```python
from build123d import *

# Parameters (mm, degrees)
F1_R = 6.35


with BuildPart() as f2:
    # F2: sweep along a path in F0
    with BuildLine(Plane.XZ) as f2_path:
        Line((-51.7302755781, 114.3), (-34.3931889452, 140.4537514452))
        ThreePointArc((-34.3931889452, 140.4537514452), (-43.0445729181, 164.4248458133), (-63.5, 149.225))
        Line((-63.5, 149.225), (-63.5, -19.05))
        ThreePointArc((-63.5, -19.05), (-31.75, -50.8), (0, -19.05))
        Line((0, -19.05), (0, 0))
    # F1 (on Top) → F2 (sweep)
    with BuildSketch(Plane.XY):
        Circle(F1_R)
    sweep(path=f2_path.line)


solid = f2.part
```
Build history of the part. All positions in model axes, mm. Coordinates: 2 decimals unless noted, no trailing zeros. Order: outer loops, then holes, each group sorted by start corner. A loop starts at its lowest first (then second) coordinate and runs counter-clockwise, first axis right, second up. Notation, with made-up numbers: (20, 4.5) -> (62, 4.5) arc R18 ccw to (62, 31.5) -> close; hole circle Ø7 at (48, 1.5). An arc over 180 degrees is marked (long way). Answer in a Markdown table with one row per item. Add a question column.
Q1. Band-saw the part on A-A, the plane z = 55. List the corners of the cut face in (x, y).
Q2. Drop flat-ended pins along their axis: pin 1 (1.5 mm diameter, centred on y = 3, z = 81.5, fed in from -X); pin 2 (4 mm diameter, centred on y = 4, z = 59.5, fed in from -X); pin 3 (2 mm diameter, centred on x = -43, y = -3.5, fed in from -Z). Give the stop position or say it passes through.
Q3. Band-saw the part on C-C, the plane x = -42. Give the number of separate pieces and of enclosed holes in the cut face, then the cut area to 3 significant figures.
Q4. Mould opens along Z. For faces 1 (the face through (-48.228, 0.279, 131.065)), 2 (the face through (0, 0, 0)), 3 (the face through (-51.804, 0.089, 114.349)), 4 (the face through (6.057, 1.907, -9.392)) say: +Z half, -Z half, draft (parallel to the pull), parting line (faces both ways), or undercut.
Q5. Wall check: line 1 along Z through (x, y) = (-53, -2.5); line 2 along Z through (x, y) = (-32, 4.5); line 3 along X through (y, z) = (0, 92.5). Give the ranges that are in metal, low to high. Write a range as [from, to].
Answers follow:
| question | item | result |
|---|---|---|
| 1 | outline | circle Ø12.7 at (-63.5, 0) |
| 2 | pin 1 | x = -69.44 |
| 2 | pin 2 | x = -69.53 |
| 2 | pin 3 | z = -55.01 |
| 3 | separate pieces | 3 |
| 3 | enclosed holes | 0 |
| 3 | area | 501 mm^2 |
| 4 | face 1 | undercut |
| 4 | face 2 | +Z half |
| 4 | face 3 | undercut |
| 4 | face 4 | draft |
| 5 | line 1 | [-50.05, -33.88], [115.14, 122.95], [157.7, 170.26] |
| 5 | line 2 | [-55.28, -46.32], [135.96, 162.27] |
| 5 | line 3 | [-69.85, -57.15] |
